Geometry: final body of the model. Coordinates: model frame, mm. Face numbers are marked on the shaded views. A direction names the side the tool comes from. Coordinates: 2 decimals unless noted, no trailing zeros. Loops run counter-clockwise (first coordinate to the right, second up) from the corner with the lowest first, then second, coordinate; pieces in that order, holes last. Notation, with made-up numbers: (87, -36) - (105, -36) arc R26 ccw to (105, -15) - close; hole circle Ø5 at (62.5, 9.25). An arc over 180 degrees is marked (long way). Put each result on its own line as item: value. Start each with the question number.
1) Material intervals for line 1 along X through (y, z) = (-63.5, -20.25); line 2 along Y through (x, z) = (63.5, -6.75); line 3 along Z through (x, y) = (-10, -48.5), sorted ascending. Write a range as from..to.
2) Section D-D on y = -10.5. Output: boundary loops of the cut face in (x, z).
3) Contact query for flat-ended pins moving along their axis: pin 1 Ø3 at (y, z) = (11.5, -2.5) entering from +X; pin 2 Ø21 at (x, y) = (13.5, -63) entering from -Z; pin 3 Ø1 at (x, y) = (13, -42) entering from -Z. Output: stop coordinate, or through.
4) Reachability of the marked faces 1 and 2 from +Z, -Z, +X, -X, +Y, -Y: full face, straight path, thin tool, end or side. Return the list, or none.
5) Section C-C on z = -4. Output: boundary loops of the cut face in (x, y).
6) Draft query along X for the marked faces 3, 4 and 5. Return one class per face: +X half, -X half, draft (parallel to the pull), parting line (faces both ways), or undercut.
7) Section B-B on z = -28. Output: boundary loops of the cut face in (x, y).
```python
from build123d import *

# Parameters (mm, degrees)
F0_W     = 101.6
F0_H     = 101.6
F1_DEPTH = 6.35
F2_R     = 3.429
F2_R_2   = 2.54
F3_DEPTH = 12.7
F4_R     = 3.429
F5_DEPTH = 25.4
F6_R     = 2.54
F7_DEPTH = 3.175


with BuildPart() as f1:
    # F0 (on Top) → F1 (new body)
    with BuildSketch(Plane.XY):
        Rectangle(F0_W, F0_H)
    extrude(amount=-F1_DEPTH)

    # F2 (on face) → F3 (join)
    with BuildSketch(Plane.XY):
        with BuildLine():
            Line((-50.8, -50.8), (-63.5, -56.896))
            ThreePointArc((-63.5, -56.896), (-68.169733183, -68.169733183), (-56.896, -63.5))
            ThreePointArc((-56.896, -63.5), (-35.0917960505, -57.5358809514), (-12.7, -54.4372529439))
            ThreePointArc((-12.7, -54.4372529439), (-8.4860183708, -58.2406426383), (-6.35, -63.5))
            ThreePointArc((-6.35, -63.5), (0, -57.15), (6.35, -63.5))
            ThreePointArc((6.35, -63.5), (8.4860183708, -58.2406426383), (12.7, -54.4372529439))
            ThreePointArc((12.7, -54.4372529439), (35.0917960505, -57.5358809514), (56.896, -63.5))
            ThreePointArc((56.896, -63.5), (68.169733183, -68.169733183), (63.5, -56.896))
            Line((63.5, -56.896), (50.8, -50.8))
            Line((50.8, -50.8), (-50.8, -50.8))
        make_face()
        with Locations((-63.5, -63.5)):
            Circle(F2_R, mode=Mode.SUBTRACT)
        with Locations((63.5, -63.5)):
            Circle(F2_R, mode=Mode.SUBTRACT)
        with BuildLine():
            ThreePointArc((6.35, -63.5), (0, -57.15), (-6.35, -63.5))
            ThreePointArc((-6.35, -63.5), (0, -69.85), (6.35, -63.5))
        make_face()
        with Locations((0, -63.5)):
            Circle(F2_R_2, mode=Mode.SUBTRACT)
    extrude(amount=-F3_DEPTH)

    # F4 (on face) → F5 (join)
    with BuildSketch(Plane(origin=(0, 0, -12.7), x_dir=(1, 0, 0), z_dir=(0, 0, -1))):
        with BuildLine():
            ThreePointArc((-56.896, 63.5), (-68.169733183, 68.169733183), (-63.5, 56.896))
            ThreePointArc((-63.5, 56.896), (-58.830266817, 58.830266817), (-56.896, 63.5))
        make_face()
        with Locations((-63.5, 63.5)):
            Circle(F4_R, mode=Mode.SUBTRACT)
        with BuildLine():
            ThreePointArc((56.896, 63.5), (58.830266817, 58.830266817), (63.5, 56.896))
            ThreePointArc((63.5, 56.896), (68.169733183, 68.169733183), (56.896, 63.5))
        make_face()
        with Locations((63.5, 63.5)):
            Circle(F4_R, mode=Mode.SUBTRACT)
    extrude(amount=F5_DEPTH)

    # F6 (on face) → F7 (cut)
    with BuildSketch(Plane(origin=(0, 0, -12.7), x_dir=(1, 0, 0), z_dir=(0, 0, -1))):
        Polygon((2.749630657, 68.2625), (-2.749630657, 68.2625), (-5.499261314, 63.5), (-2.749630657, 58.7375), (2.749630657, 58.7375), (5.499261314, 63.5), align=None)
        with Locations((0, 63.5)):
            Circle(F6_R, mode=Mode.SUBTRACT)
    extrude(amount=-F7_DEPTH, mode=Mode.SUBTRACT)


solid = f1.part
```
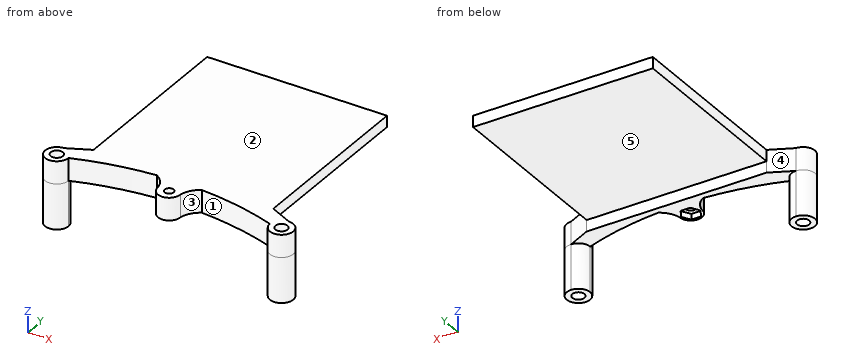
Answer block:
1. line 1: x = -70.1..-66.93, -60.07..-56.9, 56.9..60.07, 66.93..70.1
1. line 2: y = -70.1..-66.93, -60.07..-56.9
1. line 3: z = -6.35..0
2. outline: (-50.8, -6.35) - (50.8, -6.35) - (50.8, 0) - (-50.8, 0) - close
3. pin 1: stops at x = 50.8
3. pin 2: stops at z = -12.7
3. pin 3: stops at z = -6.35
4. face 1: +Z, -Z, -Y
4. face 2: +Z, +X, -X, +Y, -Y
5. outline: (-63.5, -56.9) arc R6.6 ccw (long way) to (-56.9, -63.5) arc R174.69 cw to (-12.7, -54.44) arc R12.7 cw to (-6.35, -63.5) arc R6.35 ccw to (6.35, -63.5) arc R12.7 cw to (12.7, -54.44) arc R174.69 cw to (56.9, -63.5) arc R6.6 ccw (long way) to (63.5, -56.9) - (50.8, -50.8) - (50.8, 50.8) - (-50.8, 50.8) - (-50.8, -50.8) - close; hole circle Ø6.86 at (-63.5, -63.5); hole circle Ø5.08 at (0, -63.5); hole circle Ø6.86 at (63.5, -63.5)
6. face 3: undercut
6. face 4: -X half
6. face 5: draft
7. outline: circle Ø13.21 at (-63.5, -63.5); circle Ø13.21 at (63.5, -63.5); hole circle Ø6.86 at (-63.5, -63.5); hole circle Ø6.86 at (63.5, -63.5)
